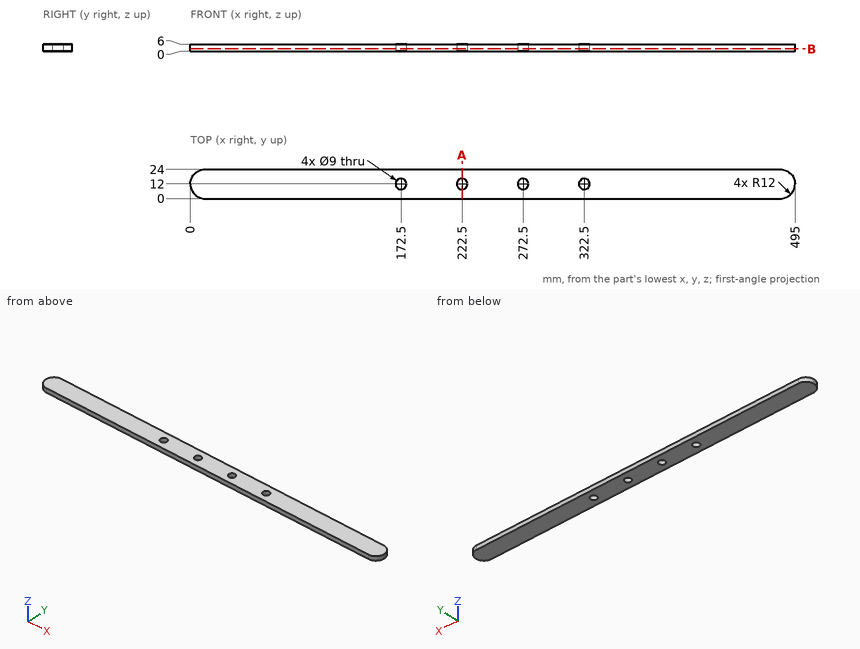
Check sheet for the drawn part. Datum: minimum x, y, z corner. Units: mm. Give positions to 0.01 mm unless a question says otherwise; leave off trailing zeros. Order: outer loops, then holes, each group sorted by start corner. A loop starts at its lowest first (then second) coordinate and runs counter-clockwise, first axis right, second up. Notation, with made-up numbers: (74, 4) - (93, 4) arc R25 ccw to (93, 20) - close; hole circle Ø2 at (60, 6). An arc over 180 degrees is marked (long way). Answer in a Markdown table with one row per item. Add a question column.
Q1. Material ranges on probe 1 along X at (y, z) = (12.5, 5.6); probe 2 along Y at (x, z) = (222.5, 4.25); probe 3 along X at (y, z) = (8, 4.55), recorded low to high. Write a range as from..to.
Q2. Gauge pin test, flat end, axial feed: pin 1 (3 mm diameter, centred on y = 8.5, z = 3.5, fed in from +X). Record the tip position at first contact, or that the pin passes through.
Q3. Cross-section at B-B, the plane z = 2.1. Count the separate pieces of the cut face and the enclosed holes in it, then the cut area to 3 significant figures.
Q4. Cross-section at A-A, the plane x = 222.5. Enter the section's corners in (y, z).
Check values:
| question | item | result |
|---|---|---|
| 1 | probe 1 | x = 0.01..168.03, 176.97..218.03, 226.97..268.03, 276.97..318.03, 326.97..494.99 |
| 1 | probe 2 | y = 0..7.5, 16.5..24 |
| 1 | probe 3 | x = 0.69..170.44, 174.56..220.44, 224.56..270.44, 274.56..320.44, 324.56..494.31 |
| 2 | pin 1 | stops at x = 494.83 |
| 3 | separate pieces | 1 |
| 3 | enclosed holes | 4 |
| 3 | area | 11,500 mm^2 |
| 4 | outline | (0, 0) - (7.5, 0) - (7.5, 6) - (0, 6) - close; (16.5, 0) - (24, 0) - (24, 6) - (16.5, 6) - close |
